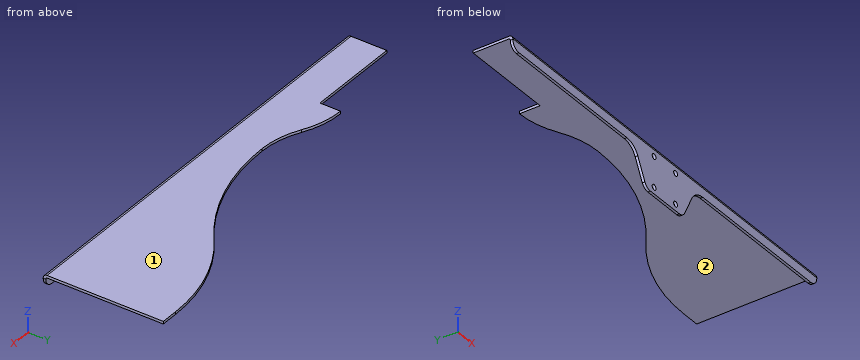
from build123d import *

# Parameters (mm, degrees)
BASIS_BLECH1_DEPTH              = 3
KANTE_LASCHE1_STRIP_W           = 15
KANTE_LASCHE1_STRIP_H           = 3
KANTE_LASCHE1_STRIP_CUT_DEPTH   = 500
KANTE_LASCHE1_DEPTH             = 500
SKIZZE19_R                      = 3.1
SCHNITT_LINEAR_AUSTRAGEN2_DEPTH = 519.20277279
SCHNITT_LINEAR_AUSTRAGEN3_DEPTH = 519.20277279
VERRUNDUNG1_R                   = 10


# Sheet-metal steps are written as plain solids
with BuildPart() as part:
    # Skizze9 → Basis-Blech1 (new body)
    with BuildSketch(Plane.XY):
        with BuildLine():
            Line((-4.107759965, 21.019858626), (495.892240035, 21.019858626))
            Line((495.892240035, 21.019858626), (495.892240035, 161.019858626))
            Line((495.892240035, 161.019858626), (475.892240035, 161.019858626))
            ThreePointArc((475.892240035, 161.019858626), (411.323644717, 150.310366837), (353.670017813, 119.328823613))
            ThreePointArc((353.670017813, 119.328823613), (281.602984183, 80.601894582), (200.892240035, 67.215029846))
            ThreePointArc((200.892240035, 67.215029846), (176.395892893, 70.261798973), (153.392240035, 79.216450312))
            ThreePointArc((153.392240035, 79.216450312), (130.388587177, 88.171101651), (105.892240035, 91.217870778))
            Line((105.892240035, 91.217870778), (105.892240035, 67.215029846))
            Line((105.892240035, 67.215029846), (-4.107759965, 67.215029846))
            Line((-4.107759965, 67.215029846), (-4.107759965, 21.019858626))
        make_face()
    extrude(amount=-BASIS_BLECH1_DEPTH)

    # Kante-Lasche1 strip (across the edge) → Kante-Lasche1 strip cut (cut)
    with BuildSketch(Plane(origin=(495.892240035, 21.019858626, -3), x_dir=(0, 1, 0), z_dir=(-1, 0, 0))):
        with Locations((-3, -1.5)):
            Rectangle(KANTE_LASCHE1_STRIP_W, KANTE_LASCHE1_STRIP_H)
    extrude(amount=KANTE_LASCHE1_STRIP_CUT_DEPTH, mode=Mode.SUBTRACT)

    # Kante-Lasche1 section (across the edge) → Kante-Lasche1 (add)
    with BuildSketch(Plane(origin=(495.892240035, 21.019858626, -3), x_dir=(0, 1, 0), z_dir=(-1, 0, 0))):
        with BuildLine():
            Line((0, 1.5), (0, 52))
            Line((0, 52), (3, 52))
            Line((3, 52), (3, 1.5))
            ThreePointArc((3, 1.5), (3.439339828, 0.439339828), (4.5, 0))
            Line((4.5, 0), (4.5, -3))
            ThreePointArc((4.5, -3), (1.318019485, -1.681980515), (0, 1.5))
        make_face()
    extrude(amount=KANTE_LASCHE1_DEPTH)

    # Skizze19 → Schnitt-Linear austragen2 (cut, through all)
    with BuildSketch(Plane.XZ.offset(-21.019858626)):
        with Locations(Location((263.569909565, -12.07233047, 0), (0, 0, 270))):
            Circle(SKIZZE19_R)
        with Locations(Location((228.214570506, -12.07233047, 0), (0, 0, 270))):
            Circle(SKIZZE19_R)
        with Locations(Location((263.569909565, -47.42766953, 0), (0, 0, 270))):
            Circle(SKIZZE19_R)
        with Locations(Location((228.214570506, -47.42766953, 0), (0, 0, 270))):
            Circle(SKIZZE19_R)
    extrude(amount=-SCHNITT_LINEAR_AUSTRAGEN2_DEPTH, mode=Mode.SUBTRACT)

    # Skizze21 → Schnitt-Linear austragen3 (cut, through all)
    with BuildSketch(Plane.XZ.offset(-21.019858626)):
        with BuildLine():
            Line((-4.107759965, -55), (-4.107759965, -15))
            Line((-4.107759965, -15), (183.53156026, -15))
            ThreePointArc((183.53156026, -15), (194.046182503, -17.986983833), (201.42010408, -26.05572809))
            Line((201.42010408, -26.05572809), (215.892240035, -55))
            Line((215.892240035, -55), (-4.107759965, -55))
        make_face()
        with BuildLine():
            Line((275.892240035, -55), (495.892240035, -55))
            Line((495.892240035, -55), (495.892240035, -15))
            Line((495.892240035, -15), (308.25291981, -15))
            ThreePointArc((308.25291981, -15), (297.738297568, -17.986983833), (290.36437599, -26.05572809))
            Line((290.36437599, -26.05572809), (275.892240035, -55))
        make_face()
    extrude(amount=-SCHNITT_LINEAR_AUSTRAGEN3_DEPTH, mode=Mode.SUBTRACT)

    # Verrundung1
    verrundung1_edges = [part.edges().sort_by_distance(p)[0] for p in [
        (275.892240035, 22.519858626, -55),
        (215.892240035, 22.519858626, -55),
        (-4.107759965, 22.519858626, -15),
        (495.892240035, 22.519858626, -15),
    ]]
    fillet(verrundung1_edges, radius=VERRUNDUNG1_R)


solid = part.part
Design review of the part built by this model. Coordinates are the model's own, in mm. Face numbers are marked on the shaded views. A direction names the side the tool comes from. Give positions to 0.01 mm unless a question says otherwise; leave off trailing zeros. Write each loop counter-clockwise with the first axis right and the second up, starting at its lowest first coordinate (ties: lowest second). Pieces come first, ordered by that corner, then holes. Notation, with made-up numbers: M 23.25,64 L 81.25,64 A19 ccw 81.25,101 Z; hole C -25.75,-38 d10. An arc over 180 degrees is marked long. Answer as a JSON object with one key per item and string values. Group by question number.
1) For line 1 along Y through (x, z) = (231, -14.5); line 2 along Z through (x, y) = (217.5, 39.5), list the stretches that pass through material, from the lowest coordinate up.
2) We need section C-C (x = 253). Give the boundary of the cut face in (y, z), and give its area (3 significant figures).
3) We need section D-D (y = 137). Give the boundary of the cut face in (x, z), and give its area (3 significant figures).
4) Tool access review of the marked faces 1 and 2: name each direction out of +Z, -Z, +X, -X, +Y, -Y from which nothing blocks a thin tool from reaching the whole face with its end or side.
5) We need section A-A (y = 73.5). Give the boundary of the cut face in (x, z).
6) Clearance check with flat-ended pins moving along their axes: pin 1 Ø10 at (x, z) = (228.21, -12.07) entering from +Y; pin 2 Ø12 at (y, z) = (135, -7) entering from -X; pin 3 Ø3.5 at (x, y) = (422.5, 23) entering from -Z; pin 4 Ø3.5 at (x, z) = (228.21, -47.43) entering from -Y (3 decimals). State where each tip first meets the part, or that it passes through.
7) We need section B-B (x = 88.5). Give the boundary of the cut face in (y, z), and give its area (3 significant figures).
Answer key:
{
 "1": {"line 1": "y = 21.02 to 24.02", "line 2": "z = -3 to 0"},
 "2": {"outline": "M 21.02,-55 L 24.02,-55 L 24.02,-4.5 A1.5 cw 25.52,-3 L 72.71,-3 L 72.71,0 L 25.52,0 A4.5 ccw 21.02,-4.5 Z", "area": "307 mm²"},
 "3": {"outline": "M 380.86,-3 L 495.89,-3 L 495.89,0 L 380.86,0 Z", "area": "345 mm²"},
 "4": {"face 1": "+Z, +X, -X, +Y, -Y", "face 2": "-Z, +X, -X, +Y"},
 "5": {"outline": "M 105.89,-3 L 166,-3 L 166,0 L 105.89,0 Z; M 256.6,-3 L 495.89,-3 L 495.89,0 L 256.6,0 Z"},
 "6": {"pin 1": "stops at y = 24.02", "pin 2": "stops at x = 369.75", "pin 3": "stops at z = -15", "pin 4": "passes through"},
 "7": {"outline": "M 21.02,-15 L 24.02,-15 L 24.02,-4.5 A1.5 cw 25.52,-3 L 67.22,-3 L 67.22,0 L 25.52,0 A4.5 ccw 21.02,-4.5 Z", "area": "171 mm²"}
}
